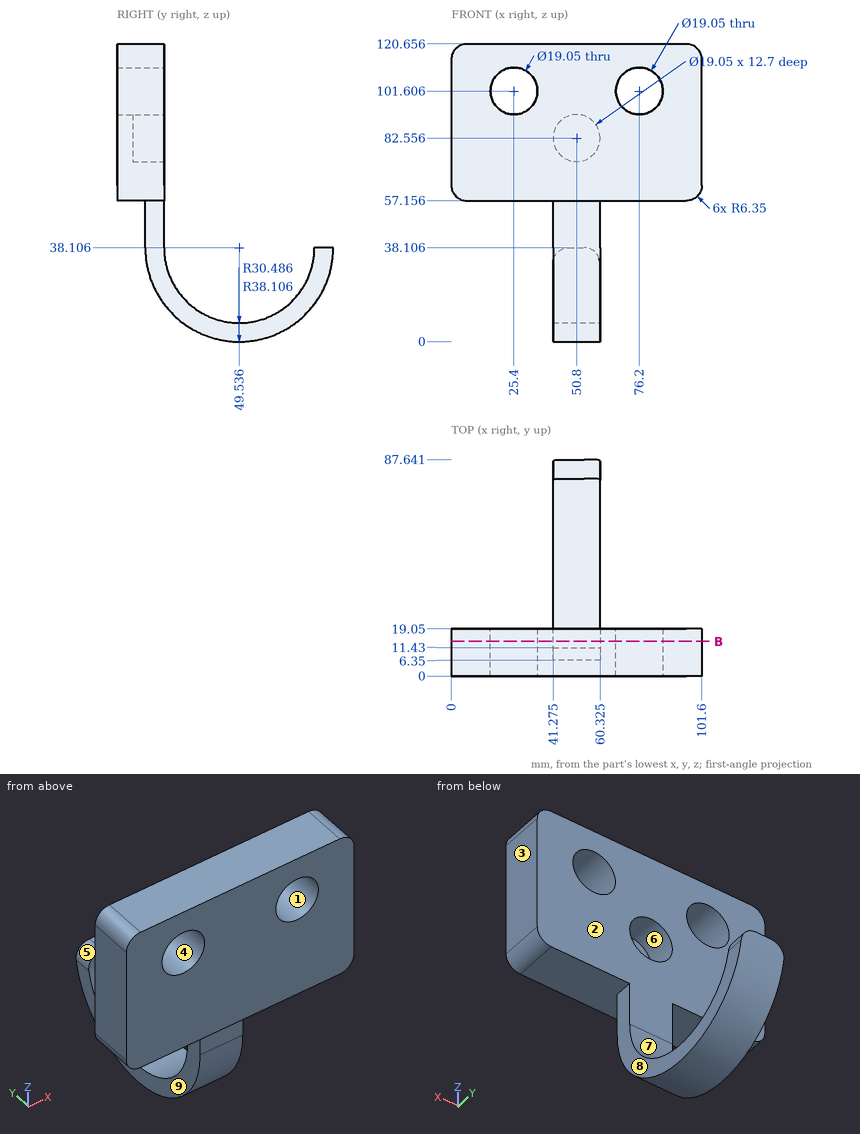
Could you check a few things on this drawing? It's one solid part, dimensions in mm from its lowest x, y, z. A direction names the side the tool comes from. Coordinates: 2 decimals unless noted, no trailing zeros. Return JSON: item names as keys, results as strings. Group by question number.
Item 1: If we section it at B-B (y = 14): Count the separate pieces of the cut face and the enclosed holes in it, then the cut area to 3 significant figures.
Item 2: Please list where these lines run through material, in increasing order: probe 1 along Z at (x, y) = (25, 11) (1 decimal); probe 2 along Z at (x, y) = (50, 10) (1 decimal); probe 3 along X at (y, z) = (16, 49) (1 decimal).
Item 3: I'm going to push flat-ended pins straight in: pin 1 Ø11.5 at (x, z) = (25.4, 101.61) entering from -Y; pin 2 Ø10 at (y, z) = (33, 12) entering from -X (3 decimals); pin 3 Ø1 at (x, y) = (43.5, 27.5) entering from +Z (1 decimal); pin 4 Ø7 at (x, y) = (52, 85) entering from +Z. Where does each tip first touch, or does it pass through?
Item 4: Which directions (+Z, -Z, +X, -X, +Y, -Y) give clear straight access to the entire face, cutting with the end or side of a thin tool? Please do the marked faces 5, 6, 7, 8 and 9.
Item 5: We'd pull the mould along X, two halves only. Please class the marked faces 1, 2, 3 and 4: pulls with the +X half, pulls with the -X half, needs draft (parallel to the pull), parting line crosses it, or undercut.
Return value:
{
 "1": {"separate pieces": "1", "enclosed holes": "3", "area": "6,190 mm^2"},
 "2": {"probe 1": "z = 57.2 to 92.1, 111.1 to 120.7", "probe 2": "z = 57.2 to 73.1, 92 to 120.7", "probe 3": "x = 41.3 to 60.3"},
 "3": {"pin 1": "passes through", "pin 2": "stops at x = 41.275", "pin 3": "stops at z = 17.6", "pin 4": "stops at z = 38.11"},
 "4": {"face 5": "+Z, -X, +Y", "face 6": "+Y", "face 7": "+Z, +X, -X", "face 8": "-Z, +X, +Y, -Y", "face 9": "-Z, -X, +Y, -Y"},
 "5": {"face 1": "undercut", "face 2": "needs draft", "face 3": "pulls with the +X half", "face 4": "undercut"}
}
